from build123d import *

# Parameters (mm, degrees)
SKETCH1_R           = 9.75
SKETCH1_R_2         = 1.25
BOSS_EXTRUDE2_DEPTH = 2
SKETCH2_W           = 8
SKETCH2_H           = 8
BOSS_EXTRUDE3_DEPTH = 24
BOSS_EXTRUDE5_START = 1.9
SKETCH7_R           = 9.75
SKETCH7_R_2         = 4.5
SKETCH7_R_3         = 1.25
BOSS_EXTRUDE5_DEPTH = 1.9
FILLET1_R           = 2.5


with BuildPart() as part:
    # Sketch1 → Boss-Extrude2 (new body)
    with BuildSketch(Plane(origin=(0, 0, 0), x_dir=(1, 0, 0), z_dir=(0, 1, 0))):
        with Locations(Location((0, 0, 0), (0, 0, 270))):
            Circle(SKETCH1_R)
        with Locations(Location((-5.78230038, 5.52856241, 0), (0, 0, 270))):
            Circle(SKETCH1_R_2, mode=Mode.SUBTRACT)
        with Locations(Location((-5.78230038, -5.52856241, 0), (0, 0, 270))):
            Circle(SKETCH1_R_2, mode=Mode.SUBTRACT)
        with Locations(Location((5.78230038, -5.52856241, 0), (0, 0, 270))):
            Circle(SKETCH1_R_2, mode=Mode.SUBTRACT)
        with Locations(Location((5.78230038, 5.52856241, 0), (0, 0, 270))):
            Circle(SKETCH1_R_2, mode=Mode.SUBTRACT)
    extrude(amount=BOSS_EXTRUDE2_DEPTH)

    # Sketch2 → Boss-Extrude3 (add)
    with BuildSketch(Plane(origin=(0, 2, 0), x_dir=(1, 0, 0), z_dir=(0, 1, 0))):
        Rectangle(SKETCH2_W, SKETCH2_H)
    extrude(amount=BOSS_EXTRUDE3_DEPTH)

    # Sketch7 → Boss-Extrude5 (add)
    with BuildSketch(Plane.XZ.offset(BOSS_EXTRUDE5_START)):
        with Locations(Location((0, 0, 0), (0, 0, 270))):
            Circle(SKETCH7_R)
        with Locations(Location((0, 0, 0), (0, 0, 90))):
            Circle(SKETCH7_R_2, mode=Mode.SUBTRACT)
        with Locations(Location((-5.78230038, 5.52856241, 0), (0, 0, 270))):
            Circle(SKETCH7_R_3, mode=Mode.SUBTRACT)
        with Locations(Location((5.78230038, 5.52856241, 0), (0, 0, 270))):
            Circle(SKETCH7_R_3, mode=Mode.SUBTRACT)
        with Locations(Location((5.78230038, -5.52856241, 0), (0, 0, 270))):
            Circle(SKETCH7_R_3, mode=Mode.SUBTRACT)
        with Locations(Location((-5.78230038, -5.52856241, 0), (0, 0, 270))):
            Circle(SKETCH7_R_3, mode=Mode.SUBTRACT)
    extrude(amount=-BOSS_EXTRUDE5_DEPTH)

    # Fillet1
    # the kernel refuses this fillet: 2.5 mm, written as the material it adds along each edge
    with BuildSketch(Plane(origin=(4, 2, -4), x_dir=(1, 0, 0), z_dir=(0, 0, 1)), Plane(origin=(-4, 2, -4), x_dir=(0, 0, -1), z_dir=(1, 0, 0)), Plane(origin=(4, 2, 4), x_dir=(0, 0, 1), z_dir=(-1, 0, 0)), Plane(origin=(-4, 2, 4), x_dir=(-1, 0, 0), z_dir=(0, 0, -1))) as fillet1_piece_1:
        with BuildLine():
            CenterArc((FILLET1_R, FILLET1_R), FILLET1_R, 180, 90)
            Line((0, FILLET1_R), (0, 0))
            Line((0, 0), (FILLET1_R, 0))
        make_face()
    extrude(amount=8)
    with BuildSketch(Plane(origin=(4, 2, -10.25), x_dir=(1, 0, 0), z_dir=(0, 0, 1))) as fillet1_piece_2a_section:
        with BuildLine():
            CenterArc((FILLET1_R, FILLET1_R), FILLET1_R, 180, 90)
            Line((0, FILLET1_R), (0, 0))
            Line((0, 0), (FILLET1_R, 0))
        make_face()
    fillet1_piece_2a = extrude(amount=14.25, mode=Mode.PRIVATE)
    fillet1_piece_2a = fillet1_piece_2a & Plane(origin=(0, 2.663763666, 0), x_dir=(0, 0, 1), z_dir=(0, -1, 0)) * Cylinder(9.75, 39, mode=Mode.PRIVATE)
    fillet1_piece_2a = fillet1_piece_2a - Plane(origin=(5.78230038, 2.663763666, -5.52856241), x_dir=(0, 0, 1), z_dir=(0, -1, 0)) * Cylinder(1.25, 39, mode=Mode.PRIVATE)
    fillet1_piece_2a = split(fillet1_piece_2a, bisect_by=Plane(origin=(4.398974619, 2.663763666, -4), z_dir=(0, 0, -1)), keep=Keep.TOP, mode=Mode.PRIVATE)
    with BuildSketch(Plane(origin=(-4, 2, -4), x_dir=(0, 0, -1), z_dir=(1, 0, 0))) as fillet1_piece_2b_section:
        with BuildLine():
            CenterArc((FILLET1_R, FILLET1_R), FILLET1_R, 180, 90)
            Line((0, FILLET1_R), (0, 0))
            Line((0, 0), (FILLET1_R, 0))
        make_face()
    fillet1_piece_2b = extrude(amount=14.25, mode=Mode.PRIVATE)
    fillet1_piece_2b = fillet1_piece_2b & Plane(origin=(0, 2.68491829, 0), x_dir=(0, 0, 1), z_dir=(0, -1, 0)) * Cylinder(9.75, 39, mode=Mode.PRIVATE)
    fillet1_piece_2b = fillet1_piece_2b - Plane(origin=(5.78230038, 2.68491829, -5.52856241), x_dir=(0, 0, 1), z_dir=(0, -1, 0)) * Cylinder(1.25, 39, mode=Mode.PRIVATE)
    fillet1_piece_2b = split(fillet1_piece_2b, bisect_by=Plane(origin=(4, 2.68491829, -4.384125447), z_dir=(1, 0, 0)), keep=Keep.TOP, mode=Mode.PRIVATE)
    fillet1_piece_2 = fillet1_piece_2a & fillet1_piece_2b
    add(fillet1_piece_2)
    with BuildSketch(Plane(origin=(10.25, 2, 4), x_dir=(0, 0, 1), z_dir=(-1, 0, 0))) as fillet1_piece_3a_section:
        with BuildLine():
            CenterArc((FILLET1_R, FILLET1_R), FILLET1_R, 180, 90)
            Line((0, FILLET1_R), (0, 0))
            Line((0, 0), (FILLET1_R, 0))
        make_face()
    fillet1_piece_3a = extrude(amount=14.25, mode=Mode.PRIVATE)
    fillet1_piece_3a = fillet1_piece_3a & Plane(origin=(0, 2.684921118, 0), x_dir=(0, 0, 1), z_dir=(0, -1, 0)) * Cylinder(9.75, 39, mode=Mode.PRIVATE)
    fillet1_piece_3a = fillet1_piece_3a - Plane(origin=(5.78230038, 2.684921118, 5.52856241), x_dir=(0, 0, 1), z_dir=(0, -1, 0)) * Cylinder(1.25, 39, mode=Mode.PRIVATE)
    fillet1_piece_3a = split(fillet1_piece_3a, bisect_by=Plane(origin=(4, 2.684921118, 4.384140978), z_dir=(1, 0, 0)), keep=Keep.TOP, mode=Mode.PRIVATE)
    with BuildSketch(Plane(origin=(4, 2, -4), x_dir=(1, 0, 0), z_dir=(0, 0, 1))) as fillet1_piece_3b_section:
        with BuildLine():
            CenterArc((FILLET1_R, FILLET1_R), FILLET1_R, 180, 90)
            Line((0, FILLET1_R), (0, 0))
            Line((0, 0), (FILLET1_R, 0))
        make_face()
    fillet1_piece_3b = extrude(amount=14.25, mode=Mode.PRIVATE)
    fillet1_piece_3b = fillet1_piece_3b & Plane(origin=(0, 2.663763629, 0), x_dir=(0, 0, 1), z_dir=(0, -1, 0)) * Cylinder(9.75, 39, mode=Mode.PRIVATE)
    fillet1_piece_3b = fillet1_piece_3b - Plane(origin=(5.78230038, 2.663763629, 5.52856241), x_dir=(0, 0, 1), z_dir=(0, -1, 0)) * Cylinder(1.25, 39, mode=Mode.PRIVATE)
    fillet1_piece_3b = split(fillet1_piece_3b, bisect_by=Plane(origin=(4.398975598, 2.663763629, 4), z_dir=(0, 0, 1)), keep=Keep.TOP, mode=Mode.PRIVATE)
    fillet1_piece_3 = fillet1_piece_3a & fillet1_piece_3b
    add(fillet1_piece_3)
    with BuildSketch(Plane(origin=(-4, 2, 4), x_dir=(-1, 0, 0), z_dir=(0, 0, -1))) as fillet1_piece_4a_section:
        with BuildLine():
            CenterArc((FILLET1_R, FILLET1_R), FILLET1_R, 180, 90)
            Line((0, FILLET1_R), (0, 0))
            Line((0, 0), (FILLET1_R, 0))
        make_face()
    fillet1_piece_4a = extrude(amount=14.25, mode=Mode.PRIVATE)
    fillet1_piece_4a = fillet1_piece_4a & Plane(origin=(0, 2.663765474, 0), x_dir=(0, 0, 1), z_dir=(0, -1, 0)) * Cylinder(9.75, 39, mode=Mode.PRIVATE)
    fillet1_piece_4a = fillet1_piece_4a - Plane(origin=(-5.78230038, 2.663765474, -5.52856241), x_dir=(0, 0, 1), z_dir=(0, -1, 0)) * Cylinder(1.25, 39, mode=Mode.PRIVATE)
    fillet1_piece_4a = split(fillet1_piece_4a, bisect_by=Plane(origin=(-4.39896904, 2.663765474, -4), z_dir=(0, 0, -1)), keep=Keep.TOP, mode=Mode.PRIVATE)
    with BuildSketch(Plane(origin=(-10.25, 2, -4), x_dir=(0, 0, -1), z_dir=(1, 0, 0))) as fillet1_piece_4b_section:
        with BuildLine():
            CenterArc((FILLET1_R, FILLET1_R), FILLET1_R, 180, 90)
            Line((0, FILLET1_R), (0, 0))
            Line((0, 0), (FILLET1_R, 0))
        make_face()
    fillet1_piece_4b = extrude(amount=14.25, mode=Mode.PRIVATE)
    fillet1_piece_4b = fillet1_piece_4b & Plane(origin=(0, 2.684918127, 0), x_dir=(0, 0, 1), z_dir=(0, -1, 0)) * Cylinder(9.75, 39, mode=Mode.PRIVATE)
    fillet1_piece_4b = fillet1_piece_4b - Plane(origin=(-5.78230038, 2.684918127, -5.52856241), x_dir=(0, 0, 1), z_dir=(0, -1, 0)) * Cylinder(1.25, 39, mode=Mode.PRIVATE)
    fillet1_piece_4b = split(fillet1_piece_4b, bisect_by=Plane(origin=(-4, 2.684918127, -4.384124985), z_dir=(-1, 0, 0)), keep=Keep.TOP, mode=Mode.PRIVATE)
    fillet1_piece_4 = fillet1_piece_4a & fillet1_piece_4b
    add(fillet1_piece_4)
    with BuildSketch(Plane(origin=(-4, 2, 10.25), x_dir=(-1, 0, 0), z_dir=(0, 0, -1))) as fillet1_piece_5a_section:
        with BuildLine():
            CenterArc((FILLET1_R, FILLET1_R), FILLET1_R, 180, 90)
            Line((0, FILLET1_R), (0, 0))
            Line((0, 0), (FILLET1_R, 0))
        make_face()
    fillet1_piece_5a = extrude(amount=14.25, mode=Mode.PRIVATE)
    fillet1_piece_5a = fillet1_piece_5a & Plane(origin=(0, 2.66376539, 0), x_dir=(0, 0, 1), z_dir=(0, -1, 0)) * Cylinder(9.75, 39, mode=Mode.PRIVATE)
    fillet1_piece_5a = fillet1_piece_5a - Plane(origin=(-5.78230038, 2.66376539, 5.52856241), x_dir=(0, 0, 1), z_dir=(0, -1, 0)) * Cylinder(1.25, 39, mode=Mode.PRIVATE)
    fillet1_piece_5a = split(fillet1_piece_5a, bisect_by=Plane(origin=(-4.398969268, 2.66376539, 4), z_dir=(0, 0, 1)), keep=Keep.TOP, mode=Mode.PRIVATE)
    with BuildSketch(Plane(origin=(4, 2, 4), x_dir=(0, 0, 1), z_dir=(-1, 0, 0))) as fillet1_piece_5b_section:
        with BuildLine():
            CenterArc((FILLET1_R, FILLET1_R), FILLET1_R, 180, 90)
            Line((0, FILLET1_R), (0, 0))
            Line((0, 0), (FILLET1_R, 0))
        make_face()
    fillet1_piece_5b = extrude(amount=14.25, mode=Mode.PRIVATE)
    fillet1_piece_5b = fillet1_piece_5b & Plane(origin=(0, 2.684921922, 0), x_dir=(0, 0, 1), z_dir=(0, -1, 0)) * Cylinder(9.75, 39, mode=Mode.PRIVATE)
    fillet1_piece_5b = fillet1_piece_5b - Plane(origin=(-5.78230038, 2.684921922, 5.52856241), x_dir=(0, 0, 1), z_dir=(0, -1, 0)) * Cylinder(1.25, 39, mode=Mode.PRIVATE)
    fillet1_piece_5b = split(fillet1_piece_5b, bisect_by=Plane(origin=(-4, 2.684921922, 4.384144633), z_dir=(-1, 0, 0)), keep=Keep.TOP, mode=Mode.PRIVATE)
    fillet1_piece_5 = fillet1_piece_5a & fillet1_piece_5b
    add(fillet1_piece_5)


solid = part.part
Here's how the part is built. I have some questions about the finished solid (model axes, mm). A direction names the side the tool comes from. Give positions to 0.01 mm unless a question says otherwise; leave off trailing zeros. Order: outer loops, then holes, each group sorted by start corner. A loop starts at its lowest first (then second) coordinate and runs counter-clockwise, first axis right, second up. Notation, with made-up numbers: (65, 24) -> (120, 24) arc R19 ccw to (120, 52) -> close; hole circle Ø1 at (78, 42.5). An arc over 180 degrees is marked (long way). Use a Markdown table: item, result. Add a question column.
Item 1: Imagine slicing it at D-D on y = 6. Please give me the cut outline in (x, z), plus the area to 3 significant figures.
Item 2: Imagine slicing it at B-B on z = 0. Please give me the cut outline in (x, y).
Item 3: Will these pins go through, and if not, where does the flat tip stop? pin 1 (1.5 mm diameter, centred on x = 5, z = -4, fed in from +Y); pin 2 (2.5 mm diameter, centred on y = 16, z = 1.5, fed in from -X); pin 3 (2 mm diameter, centred on x = -4.5, z = -6.5, fed in from +Y).
Item 4: For faces 4 (the face through (-4, 15, 0)), 5 (the face through (0, 15, 4)), 6 (the face through (-1.352, -0.963, 4.292)), which set-ups out of +Z, -Z, +X, -X, +Y, -Y let a thin tool reach every point of the face, with its end or its side?
Item 5: I need wall thicknesses on line 1 (X direction, y = -1.45, z = 0); line 2 (X direction, y = 6, z = 2). Which ranges of each line are inside material? Lowest first, please.
Item 6: Imagine slicing it at C-C on z = 5.5. Please give me the cut outline in (x, y), plus the area to 3 significant figures.
Item 7: If we mould it in two halves opening along X, with no side actions, what happens to faces 1 (the face through (0, 0, 0)), 2 (the face through (4.713, 2.752, -0.067)), 3 (the face through (0, 26, 0))? For each: pulls with the +X half, pulls with the -X half, needs draft (parallel to the pull), parting line crosses it, or undercut.
Item 8: Imagine slicing it at A-A on x = 0. Please give me the cut outline in (y, z), plus the area to 3 significant figures.
Data:
| question | item | result |
|---|---|---|
| 1 | outline | (-4, -4) -> (4, -4) -> (4, 4) -> (-4, 4) -> close |
| 1 | area | 64.0 mm² |
| 2 | outline | (-9.75, -1.9) -> (-4.5, -1.9) -> (-4.5, 0) -> (4.5, 0) -> (4.5, -1.9) -> (9.75, -1.9) -> (9.75, 2) -> (6.5, 2) arc R2.5 cw to (4, 4.5) -> (4, 26) -> (-4, 26) -> (-4, 4.5) arc R2.5 cw to (-6.5, 2) -> (-9.75, 2) -> close |
| 3 | pin 1 | stops at y = 3.41 |
| 3 | pin 2 | stops at x = -4 |
| 3 | pin 3 | stops at y = 2.21 |
| 4 | face 4 | +Z, -Z, -X, +Y |
| 4 | face 5 | +Z, +X, -X, +Y |
| 4 | face 6 | -Y |
| 5 | line 1 | x = -9.75 to -4.5, 4.5 to 9.75 |
| 5 | line 2 | x = -4 to 4 |
| 6 | outline | (-8.05, -1.9) -> (-7.03, -1.9) -> (-7.03, 2) -> (-8.05, 2) -> close; (-4.53, -1.9) -> (4.53, -1.9) -> (4.53, 2.21) -> (-4.53, 2.21) -> close; (7.03, -1.9) -> (8.05, -1.9) -> (8.05, 2) -> (7.03, 2) -> close |
| 6 | area | 45.2 mm² |
| 7 | face 1 | undercut |
| 7 | face 2 | pulls with the +X half |
| 7 | face 3 | needs draft |
| 8 | outline | (-1.9, -9.75) -> (2, -9.75) -> (2, -6.5) arc R2.5 cw to (4.5, -4) -> (26, -4) -> (26, 4) -> (4.5, 4) arc R2.5 cw to (2, 6.5) -> (2, 9.75) -> (-1.9, 9.75) -> (-1.9, 4.5) -> (0, 4.5) -> (0, -4.5) -> (-1.9, -4.5) -> close |
| 8 | area | 254 mm² |
